from build123d import *

# Parameters (mm, degrees)
SKETCH_1_R          = 2
EXTRUDE_1_DEPTH     = 30
SKETCH_3_W          = 4.2
SKETCH_3_H          = 1
CUT_EXTRUDE_1_DEPTH = 8
CUT_EXTRUDE_2_REACH = 32.256
SKETCH_4_W          = 1
SKETCH_4_H          = 4
SKETCH_6_W          = 4.2
SKETCH_6_H          = 1
CUT_EXTRUDE_3_DEPTH = 8
SKETCH_7_W          = 1
SKETCH_7_H          = 4
CUT_EXTRUDE_4_DEPTH = 31.255619313


with BuildPart() as part:
    # 草图1 → 凸台-拉伸1 (new body)
    with BuildSketch(Plane.XY):
        Circle(SKETCH_1_R)
    extrude(amount=-EXTRUDE_1_DEPTH)

    # 草图2 → 旋转1 (revolve)
    with BuildSketch(Plane(origin=(0, 0, 0), x_dir=(1, 0, 0), z_dir=(0, 1, 0))):
        Polygon((0, 0), (0, 2), (2.2, 2), (2, 0), align=None)
    revolve(axis=Axis((0, 0, 0), (0, 0, -1)))

    # 草图3 → 切除-拉伸1 (cut)
    with BuildSketch(Plane.XY):
        with Locations((0, 1.75)):
            Rectangle(SKETCH_3_W, SKETCH_3_H)
        with Locations((0, -1.75)):
            Rectangle(SKETCH_3_W, SKETCH_3_H)
    extrude(amount=-CUT_EXTRUDE_1_DEPTH, mode=Mode.SUBTRACT)

    # 草图4 → 切除-拉伸2 (cut, up to next)
    with BuildSketch(Plane.XZ.offset(1.25), mode=Mode.PRIVATE) as cut_extrude_2_sk1:
        with Locations((0, -2)):
            Rectangle(SKETCH_4_W, SKETCH_4_H)
    cut_extrude_2_tool1 = extrude(cut_extrude_2_sk1.sketch, amount=-CUT_EXTRUDE_2_REACH, mode=Mode.PRIVATE) & part.part
    add(cut_extrude_2_tool1.solids().sort_by_distance((0, -1.25, -2))[0], mode=Mode.SUBTRACT)

    # 草图5 → 旋转2 (revolve)
    with BuildSketch(Plane(origin=(0, 0, 0), x_dir=(1, 0, 0), z_dir=(0, 1, 0))):
        Polygon((0, 30), (0, 28), (2.2, 28), (2, 30), align=None)
    revolve(axis=Axis((0, 0, -58.137689197), (0, 0, -1)))

    # 草图6 → 切除-拉伸3 (cut)
    with BuildSketch(Plane(origin=(0, 0, -30), x_dir=(-1, 0, 0), z_dir=(0, 0, -1))):
        with Locations((0, 1.75)):
            Rectangle(SKETCH_6_W, SKETCH_6_H)
        with Locations((0, -1.75)):
            Rectangle(SKETCH_6_W, SKETCH_6_H)
    extrude(amount=-CUT_EXTRUDE_3_DEPTH, mode=Mode.SUBTRACT)

    # 草图7 → 切除-拉伸4 (cut, through all)
    with BuildSketch(Plane(origin=(0, 1.25, 0), x_dir=(1, 0, 0), z_dir=(0, 1, 0))):
        with Locations((0, 28)):
            Rectangle(SKETCH_7_W, SKETCH_7_H)
    extrude(amount=-CUT_EXTRUDE_4_DEPTH, mode=Mode.SUBTRACT)


solid = part.part
Here's how the part is built. I have some questions about the finished solid (model axes, mm). A direction names the side the tool comes from. Coordinates: 2 decimals unless noted, no trailing zeros. Order: outer loops, then holes, each group sorted by start corner. A loop starts at its lowest first (then second) coordinate and runs counter-clockwise, first axis right, second up. Notation, with made-up numbers: M -22.75,-27 L 2.25,-27 A18 cw 2.25,2 Z; hole C 66,56.25 d9. An arc over 180 degrees is marked long. Answer as CSV lines item,"result". Start each with the question number.
1. I need wall thicknesses on line 1 (Z direction, x = 0.05, y = -0.65); line 2 (Z direction, x = -0.55, y = -1.4); line 3 (X direction, y = 0.65, z = -26.5). Which ranges of each line are inside material? Lowest first, please. Write a range as [from, to].
2. I want a section at A-A, the plane y = 0. Write out the boundary of the cut face in (x, z), and give its area (3 significant figures).
3. We'd pull the mould along X, two halves only. Please class faces 5 (the flat face through (0, 1.25, -25)), 6 (the conical face through (-2.1, 0, -29)), 7 (the flat face through (0, 0, -4)): released by +X, released by -X, zero draft, split by the parting line, or undercut.
4. I want a section at B-B, the plane x = 0. Write out the boundary of the cut face in (y, z).
5. I want a section at D-D, the plane x = -1.1. Write out the boundary of the cut face in (y, z).
6. I want a section at C-C, the plane z = -18.5. Write out the boundary of the cut face in (x, y), and give its area (3 significant figures).
7. For pin 1 (0.6 mm diameter, centred on x = -0.5, y = 2, fed in from +Z); pin 2 (1.2 mm diameter, centred on y = 0.5, z = -27, fed in from +X); pin 3 (2 mm diameter, centred on x = 1, z = -6, fed in from -Y), each with a flat end and sliding along its axis, tell me the tip position at first contact or that it passes through.
8. On a 3-axis mill with a long thin cutter (end or side, diameter ignored), from which of +Z, -Z, +X, -X, +Y, -Y can I reach the whole of each face in a straight line? I mean faces 1 (the flat face through (-0.5, 0, -28)), 2 (the flat face through (0.5, 0, -2)), 3 (the flat face through (0, -1.25, -25)), 4 (the flat face through (0, -1.25, -5)). Say none if no direction works.
Recorded:
1,line 1,"z = [-26, -4]"
1,line 2,"z = [-22, -8]"
1,line 3,"x = [-1.89, -0.5], [0.5, 1.89]"
2,outline,"M -2.2,-28 L -2,-30 L -0.5,-30 L -0.5,-26 L 0.5,-26 L 0.5,-30 L 2,-30 L 2.2,-28 L 2,-28 L 2,-2 L 2.2,-2 L 2,0 L 0.5,0 L 0.5,-4 L -0.5,-4 L -0.5,0 L -2,0 L -2.2,-2 L -2,-2 L -2,-28 Z"
2,area,"113 mm2"
3,face 5,"zero draft"
3,face 6,"released by -X"
3,face 7,"undercut"
4,outline,"M -2,-22 L -1.25,-22 L -1.25,-26 L 1.25,-26 L 1.25,-22 L 2,-22 L 2,-8 L 1.25,-8 L 1.25,-4 L -1.25,-4 L -1.25,-8 L -2,-8 Z"
5,outline,"M -1.67,-22 L -1.25,-22 L -1.25,-30 L 1.25,-30 L 1.25,-22 L 1.67,-22 L 1.67,-8 L 1.25,-8 L 1.25,0 L -1.25,0 L -1.25,-8 L -1.67,-8 Z"
6,outline,"C 0,0 d4"
6,area,"12.6 mm2"
7,pin 1,"stops at z = -8"
7,pin 2,"stops at x = 2"
7,pin 3,"stops at y = -1.25"
8,face 1,"-Z, +Y, -Y"
8,face 2,"+Z, +Y, -Y"
8,face 3,"-Z, +X, -X, -Y"
8,face 4,"+Z, +X, -X, -Y"
